Verification items for the finished model (mm, model axes). A direction names the side the tool comes from. Give positions to 0.01 mm unless a question says otherwise; leave off trailing zeros. Loops run counter-clockwise (first coordinate to the right, second up) from the corner with the lowest first, then second, coordinate; pieces in that order, holes last. Notation, with made-up numbers: M 74.5,46 L 117.5,46 A16 cw 117.5,73 Z; hole C 60.25,15.5 d11. An arc over 180 degrees is marked long. Answer in a Markdown table with one row per item.
```python
from build123d import *

# Parameters (mm, degrees)
SKETCH1_W           = 50.8
SKETCH1_H           = 25.4
BOSS_EXTRUDE1_DEPTH = 304.8
FILLET1_R           = 25.4
CUT_EXTRUDE1_DEPTH  = 311.04651264
FILLET2_R           = 254
SKETCH7_R           = 3.175
CUT_EXTRUDE2_DEPTH  = 311.04651264
CUT_EXTRUDE3_DEPTH  = 311.04651264


with BuildPart() as part:
    # Sketch1 → Boss-Extrude1 (new body)
    with BuildSketch(Plane.XY):
        with Locations((-25.4, 12.7)):
            Rectangle(SKETCH1_W, SKETCH1_H)
    extrude(amount=BOSS_EXTRUDE1_DEPTH)

    # Fillet1
    fillet1_edges = [part.edges().sort_by_distance(p)[0] for p in [
        (0, 12.7, 304.8),
        (-50.8, 12.7, 304.8),
    ]]
    fillet(fillet1_edges, radius=FILLET1_R - 0.0001)  # a hair under: the kernel refuses the full size

    # Sketch6 → Cut-Extrude1 (cut, through all)
    with BuildSketch(Plane(origin=(0, 25.4, 0), x_dir=(1, 0, 0), z_dir=(0, 1, 0))):
        Polygon((-50.8, 0), (0, -87.988181024), (0, 0), align=None)
    extrude(amount=-CUT_EXTRUDE1_DEPTH, mode=Mode.SUBTRACT)

    # Fillet2
    fillet2_edges = [part.edges().sort_by_distance(p)[0] for p in [
        (0, 12.7, 87.988181024),
    ]]
    fillet(fillet2_edges, radius=FILLET2_R)

    # Sketch7 → Cut-Extrude2 (cut, through all)
    with BuildSketch(Plane(origin=(0, 25.4, 0), x_dir=(1, 0, 0), z_dir=(0, 1, 0))):
        with Locations(Location((-25.4, -279.4, 0), (0, 0, 180))):
            Circle(SKETCH7_R)
    extrude(amount=-CUT_EXTRUDE2_DEPTH, mode=Mode.SUBTRACT)

    # Sketch8 → Cut-Extrude3 (cut, through all)
    with BuildSketch(Plane(origin=(0, 25.4, 0), x_dir=(1, 0, 0), z_dir=(0, 1, 0))):
        with BuildLine():
            Line((-27.305, -247.65), (-27.305, -222.25))
            ThreePointArc((-27.305, -222.25), (-25.4, -220.345), (-23.495, -222.25))
            Line((-23.495, -222.25), (-23.495, -247.65))
            ThreePointArc((-23.495, -247.65), (-25.4, -249.555), (-27.305, -247.65))
        make_face()
    extrude(amount=-CUT_EXTRUDE3_DEPTH, mode=Mode.SUBTRACT)


solid = part.part
```
Item 1: Sectioned sample at C-C (x = -14). Record the cut outline in (y, z).
Reported:
| item | result |
|---|---|
| outline | M 0,72.88 L 25.4,72.88 L 25.4,302.1 L 0,302.1 Z |
Item 2: Release check for a two-part mould opening along Z. For faces 3 (the flat face through (-26, 25.4, 184)), 4 (the flat face through (-23.495, 13, 235)), 5 (the cylindrical face through (-7.24, 12.88, 297.16)) record: released by +Z, released by -Z, zero draft, split by the parting line, or undercut.
Reported:
| item | result |
|---|---|
| face 3 | zero draft |
| face 4 | undercut |
| face 5 | released by +Z |
Item 3: Go/stop test with a flat-tipped pin: pin 1 (12 mm diameter, centred on x = -29, y = 9.5, fed in from -Z). Record where the tip stops, or that it passes through.
Reported:
| item | result |
|---|---|
| pin 1 | stops at z = 27.37 |
Item 4: Scan lines: L1, parallel to X at y = 6.5, z = 279.4 (3 decimals); L2, parallel to Z at x = -25.4, y = 16 (3 decimals); L3, parallel to X at y = 1.75, z = 240 (3 decimals). Record each from-to range of solid material in increasing order. Write a range as [from, to].
Reported:
| item | result |
|---|---|
| L1 | x = [-50.8, -28.575], [-22.225, 0] |
| L2 | z = [45.331, 220.345], [249.555, 276.225], [282.575, 304.8] |
| L3 | x = [-50.8, -27.305], [-23.495, 0] |
Item 5: Sectioned sample at A-A (y = 18.5). State how many separate pieces and enclosed holes the cut face has, and give its area (3 significant figures).
Reported:
| item | result |
|---|---|
| separate pieces | 1 |
| enclosed holes | 2 |
| area | 12,400 mm^2 |
Item 6: Tool access check on faces 1 (the cylindrical face through (-8.9, 12.5, 89.4)), 2 (the flat face through (-27.305, 13, 235)). Record the directions out of +Z, -Z, +X, -X, +Y, -Y that give a thin tool (end or side, any length) a straight path to the whole face; none if there is none.
Reported:
| item | result |
|---|---|
| face 1 | -Z, +X, +Y, -Y |
| face 2 | +Y, -Y |
Item 7: Sectioned sample at B-B (z = 56.5). Record the cut outline in (x, y), and give its area (3 significant figures).
Reported:
| item | result |
|---|---|
| outline | M -50.8,0 L -20.32,0 L -20.32,25.4 L -50.8,25.4 Z |
| area | 774 mm^2 |
